The listing builds one solid part. Answer for the finished solid, in the listing's coordinates (mm). Face numbers are marked on the shaded views. A direction names the side the tool comes from. Coordinates: 2 decimals unless noted, no trailing zeros. Order: outer loops, then holes, each group sorted by start corner. A loop starts at its lowest first (then second) coordinate and runs counter-clockwise, first axis right, second up. Notation, with made-up numbers: M 77,39.25 L 93,39.25 A20 ccw 93,43.25 Z; hole C -38.75,41.5 d10. An arc over 180 degrees is marked long. One line per item, written item: value. Start each with the question number.
Q1. Straight lines are drawn through the part: line 1 along Z through (x, y) = (19, -7.25); line 2 along X through (y, z) = (-7.25, 44.5); line 3 along Y through (x, z) = (-19, 59). For each, find the intervals that lie inside material, in ascending order. Write a range as [from, to].
Q2. Determine the mould class of the marked faces 3, 4, 5 and 6 for opening direction X: pulls with the +X half, pulls with the -X half, needs draft (parallel to the pull), parting line crosses it, or undercut.
Q3. For the marked faces 1 and 2, determine the directions among +Z, -Z, +X, -X, +Y, -Y from which every point of the face is accessible in a straight line to the end or side of a thin tool.
Q4. The part is cut by section C-C on z = 24. Give the vertices of the cut face in (x, y), then the cut area to 3 significant figures.
Q5. Each of these flat-tipped pins is pushed along its axis until it touches: pin 1 Ø2 at (x, z) = (25, 89.5) entering from -Y; pin 2 Ø0.8 at (x, z) = (2, 89.5) entering from -Y. Where does it stop, or does it pass through?
Q6. The part is cut by section B-B on y = -14.25. Give the vertices of the cut face in (x, z), then the cut area to 3 significant figures.
Q7. The part is cut by section A-A on x = 18.5. Give the vertices of the cut face in (y, z) (3 decimals).
Solid Edge part; units mm, degrees
sketch "Sketch1" plane through (0, 0, 0) normal (0, -1, 0) x (1, 0, 0)
  line L0 (-38.5, 90.2089) -> (-38.5, -79.7911)
  line L1 (-38.5, -79.7911) -> (41.5, -79.7911)
  line L2 (41.5, -79.7911) -> (41.5, 90.2089)
  line L3 (41.5, 90.2089) -> (-38.5, 90.2089)
extrude "Protrusion1" add sketch "Sketch1" along normal blind 18
sketch "Sketch2" plane through (1.5, -18, 5.2089) normal (0, -1, 0) x (1, 0, 0)
  line L0 (35.5, -82.7405) -> (35.5, 82.2595)
  line L1 (35.5, 82.2595) -> (-38.5, 82.2595)
  line L2 (-38.5, 82.2595) -> (-38.5, -82.7405)
  line L3 (-38.5, -82.7405) -> (35.5, -82.7405)
extrude "ExtrudedCutout_1" cut sketch "Sketch2" against normal blind 16.2133
sketch "Sketch3" plane through (1.5, 0, 5.2089) normal (0, 1, 0) x (0, 0, 1)
  line L0 (-81.6739, 0.5403) -> (-81.6739, 34.5403)
  line L1 (-81.6739, 34.5403) -> (-41.6739, 34.5403)
  line L2 (-41.6739, 34.5403) -> (-41.6739, 0.5403)
  line L3 (-41.6739, 0.5403) -> (-81.6739, 0.5403)
extrude "Cutout1" cut sketch "Sketch3" against normal up to next
fillet "Round_1" radius 2 7 edges at (-38.5, -18, 5.2089) (41.5, -18, 5.2089) (1.5, 0, -79.7911) (1.5, -18, 90.2089) (41.5, 0, 5.2089) (-38.5, 0, 5.2089) (1.5, 0, 90.2089)
sketch "Sketch4" plane through (41.5, -9, 5.2089) normal (1, 0, 0) x (0, 0, -1)
  line L0 (67.8445, -2.0423) -> (67.8445, 2.9577)
  line L1 (67.8445, 2.9577) -> (30.8445, 2.9577)
  line L2 (30.8445, 2.9577) -> (30.8445, -2.0423)
  line L3 (30.8445, -2.0423) -> (67.8445, -2.0423)
extrude "Cutout2" cut sketch "Sketch4" against normal up to next
sketch "Sketch5" plane through (41.5, -9, 5.2089) normal (1, 0, 0) x (0, 0, -1)
  line L0 (-4.7818, 2.9577) -> (-4.7818, -2.0423)
  line L1 (-4.7818, -2.0423) -> (12.8445, -2.0423)
  line L2 (12.8445, -2.0423) -> (12.8445, 2.9577)
  line L3 (12.8445, 2.9577) -> (-4.7818, 2.9577)
extrude "Cutout3" cut sketch "Sketch5" against normal up to next
sketch "Sketch6" plane through (1.5, -9, 90.2089) normal (0, 0, 1) x (1, 0, 0)
  circle A0 centre (-25.6335, 1) radius 2
extrude "Cutout4" cut sketch "Sketch6" along normal up to next and the other way up to next
sketch "Sketch7" plane through (-14.2035, -9.0953, 90.2089) normal (0, 0, 1) x (1, 0, 0)
  line L0 (0, 2) -> (4, 2)
  line L1 (4, 2) -> (4, 0)
  line L2 (4, 0) -> (0, 0)
  line L3 (0, 0) -> (0, 2)
extrude "Cutout5" cut sketch "Sketch7" against normal up to next
sketch "Sketch8" plane through (1.5, -9, 90.2089) normal (0, 0, 1) x (1, 0, 0)
  line L0 (-1.9412, -0.0953) -> (-1.9412, 1.9047)
  line L1 (-1.9412, 1.9047) -> (8.0588, 1.9047)
  line L2 (8.0588, 1.9047) -> (8.0588, -0.0953)
  line L3 (8.0588, -0.0953) -> (-1.9412, -0.0953)
extrude "Cutout6" cut sketch "Sketch8" against normal up to next
sketch "Sketch9" plane through (1.5, -9, 90.2089) normal (0, 0, 1) x (1, 0, 0)
  line L0 (20.0588, 1.9909) -> (20.0588, -0.0091)
  line L1 (20.0588, -0.0091) -> (30.8058, -0.0091)
  line L2 (30.8058, -0.0091) -> (30.8058, 1.9909)
  line L3 (30.8058, 1.9909) -> (20.0588, 1.9909)
extrude "Cutout7" cut sketch "Sketch9" against normal up to next
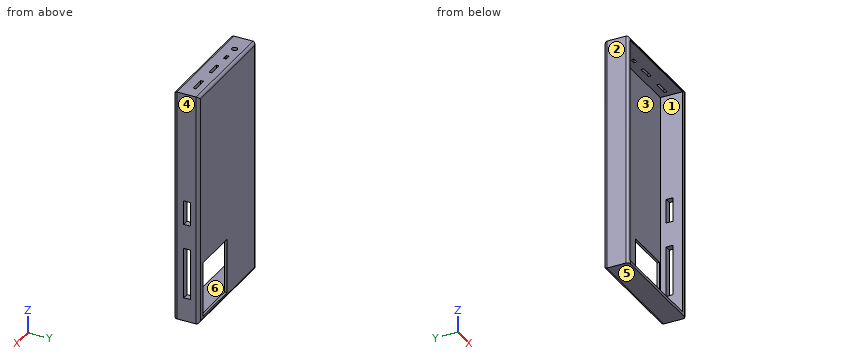
Output:
1. line 1: z = [-79.79, -77.53], [87.47, 90.21]
1. line 2: x = [-38.5, -37], [37, 41.5]
1. line 3: y = [-1.79, 0]
2. face 3: undercut
2. face 4: pulls with the +X half
2. face 5: needs draft
2. face 6: undercut
3. face 1: -Y
3. face 2: +Z, -Z, -X, +Y, -Y
4. outline: M -38.5,-16 A2 ccw -37,-17.94 L -37,-1.79 L 37,-1.79 L 37,-18 L 39.5,-18 A2 ccw 41.5,-16 L 41.5,-2 A2 ccw 39.5,0 L -36.5,0 A2 ccw -38.5,-2 Z
4. area: 237 mm^2
5. pin 1: stops at y = -17.98
5. pin 2: stops at y = -17.79
6. outline: M -38.5,-79.79 L 41.5,-79.79 L 41.5,90.21 L -38.5,90.21 Z; hole M -37,-77.53 L 37,-77.53 L 37,87.47 L -37,87.47 Z
6. area: 1,390 mm^2
7. outline: M -18,-79.791 L -2,-79.791 A2 ccw 0,-77.791 L 0,-76.465 L -1.787,-76.465 L -1.787,-77.532 L -18,-77.532 Z; M -18,87.468 L -1.787,87.468 L -1.787,-36.465 L 0,-36.465 L 0,88.209 A2 ccw -2,90.209 L -16,90.209 A2 ccw -18,88.209 Z
